```python
from build123d import *

# Parameters (mm, degrees)
F0_W     = 300
F0_H     = 107
F1_DEPTH = 20
F2_R     = 5
F3_W     = 13
F3_H     = 5
F4_DEPTH = 16.5
F5_R     = 1.8
F6_DEPTH = 4.5
F7_W     = 7
F7_H     = 12.5
F8_DEPTH = 25


with BuildPart() as f1:
    # F0 (on Top) → F1 (new body)
    with BuildSketch(Plane.XY):
        with Locations((150, 53.5)):
            Rectangle(F0_W, F0_H)
    extrude(amount=F1_DEPTH)

    # F2
    f2_edges = [f1.edges().sort_by_distance(p)[0] for p in [
        (0, 107, 10),
        (0, 0, 10),
        (300, 0, 10),
        (300, 107, 10),
    ]]
    fillet(f2_edges, radius=F2_R)

    # F3 (on face) + F1_face1 (on face) → F4 (cut)
    with BuildSketch(Plane.XY.offset(20)):
        Polygon((17.5, 102), (5, 102), (5, 5), (295, 5), (295, 102), (30.5, 102), align=None)
        with Locations((24, 104.5)):
            Rectangle(F3_W, F3_H)
    with BuildSketch(Plane(origin=(150, 53.5, 0), x_dir=(1, 0, 0), z_dir=(0, 0, -1))):
        with BuildLine():
            Line((-150, 48.5), (-150, -48.5))
            ThreePointArc((-150, -48.5), (-148.5355339059, -52.0355339059), (-145, -53.5))
            Line((-145, -53.5), (145, -53.5))
            ThreePointArc((145, -53.5), (148.5355339059, -52.0355339059), (150, -48.5))
            Line((150, -48.5), (150, 48.5))
            ThreePointArc((150, 48.5), (148.5355339059, 52.0355339059), (145, 53.5))
            Line((145, 53.5), (-145, 53.5))
            ThreePointArc((-145, 53.5), (-148.5355339059, 52.0355339059), (-150, 48.5))
        make_face()
    extrude(amount=-F4_DEPTH, dir=(0, 0, 1), mode=Mode.SUBTRACT)

    # F5 (on face) → F6 (join)
    with BuildSketch(Plane.XY.offset(3.5)):
        with Locations((269.5, 74)):
            Circle(F5_R)
        with Locations((226.4248728752, 14.5)):
            Circle(F5_R)
        with Locations((133.5, 54.5)):
            Circle(F5_R)
        with Locations((30.5, 72)):
            Circle(F5_R)
        with BuildLine():
            Line((8.6, 46.8000370503), (5, 46.8000370503))
            Line((5, 46.8000370503), (5, 43.2001111493))
            Line((5, 43.2001111493), (8.6230977842, 43.2001111493))
            ThreePointArc((8.6230977842, 43.2001111493), (10.4, 45.0115491298), (8.6, 46.8000370503))
        make_face()
        with BuildLine():
            Line((295, 43.2001111493), (295, 46.8000370503))
            Line((295, 46.8000370503), (291.4, 46.8000370503))
            ThreePointArc((291.4, 46.8000370503), (289.6, 45.0115491298), (291.3769022158, 43.2001111493))
            Line((291.3769022158, 43.2001111493), (295, 43.2001111493))
        make_face()
    extrude(amount=F6_DEPTH)

    # F7 (on face) → F8 (cut)
    with BuildSketch(Plane.XY.offset(3.5)):
        with Locations((33.5, 53.75)):
            Rectangle(F7_W, F7_H)
    extrude(amount=-F8_DEPTH, mode=Mode.SUBTRACT)


solid = f1.part
```
Work out the finished part from the listing and answer in its coordinate system (mm). A direction names the side the tool comes from. Coordinates: 2 decimals unless noted, no trailing zeros. Loops run counter-clockwise (first coordinate to the right, second up) from the corner with the lowest first, then second, coordinate; pieces in that order, holes last. Notation, with made-up numbers: M 72.25,15 L 117.25,15 A26 cw 117.25,34 Z; hole C 21,-12.75 d8. An arc over 180 degrees is marked long. Use CSV: the item, a comma, the result in double quotes. Start each with the question number.
(1) For faces 1 (the face through (11, 102, 12)), 2 (the face through (30.5, 104, 12)), 3 (the face through (105, 2, 20)), determine the directions among +Z, -Z, +X, -X, +Y, -Y from which every point of the face is accessible in a straight line to the end or side of a thin tool.
(2) Find section A-A, the plane z = 12.25. Give the vertices of the cut face in (x, y), then the cut area to 3 significant figures.
(3) For a pull along X with two mould halves and no side action, classify faces 4 (the face through (148, 5, 12)), 5 (the face through (17.5, 104, 12)), 6 (the face through (1, 105, 10)), 7 (the face through (148, 54, 0)) as +X half, -X half, draft (parallel to the pull), parting line (faces both ways), or undercut.
(4) Find section B-B, the plane x = 201.5. Give the vertices of the cut face in (y, z), then the cut area to 4 significant figures.
(5) Find section C-C, the plane y = 96. Give the vertices of the cut face in (x, z), then the cut area to 4 significant figures.
(6) Consider line 1 (Y direction, x = 265.5, z = 8.5); line 2 (X direction, y = 10.5, z = 6.5); line 3 (Y direction, x = 29.5, z = 17.5). Determine where each line is inside the solid, lowest interval first.
(7) Given pin 1 Ø3 at (x, y) = (226.5, 14.5) entering from +Z; pin 2 Ø4 at (x, y) = (42, 30) entering from +Z, each flat-ended and moving along its own axis, determine where each tip first touches the part or whether it passes through.
Recorded:
1,face 1,"+Z"
1,face 2,"+Z, +Y"
1,face 3,"+Z, +X, -X, +Y, -Y"
2,outline,"M 0,5 A5 ccw 5,0 L 295,0 A5 ccw 300,5 L 300,102 A5 ccw 295,107 L 30.5,107 L 30.5,102 L 295,102 L 295,5 L 5,5 L 5,102 L 17.5,102 L 17.5,107 L 5,107 A5 ccw 0,102 Z"
2,area,"3,880 mm^2"
3,face 4,"undercut"
3,face 5,"undercut"
3,face 6,"-X half"
3,face 7,"draft"
4,outline,"M 0,0 L 107,0 L 107,20 L 102,20 L 102,3.5 L 5,3.5 L 5,20 L 0,20 Z"
4,area,"539.5 mm^2"
5,outline,"M 0,0 L 300,0 L 300,20 L 295,20 L 295,3.5 L 5,3.5 L 5,20 L 0,20 Z"
5,area,"1,215 mm^2"
6,line 1,"y = 0 to 5, 102 to 107"
6,line 2,"x = 0 to 5, 295 to 300"
6,line 3,"y = 0 to 5"
7,pin 1,"stops at z = 8"
7,pin 2,"stops at z = 3.5"
